from build123d import *

# Parameters (mm, degrees)
ESQUISSE1_W                                       = 17
ESQUISSE1_H                                       = 40
BOSS_EXTRU_1_DEPTH                                = 4
CHAMBRAGE_POUR_VIS_SIX_PANS_CREUX_M21_D           = 2.4
CHAMBRAGE_POUR_VIS_SIX_PANS_CREUX_M21_CBORE_D     = 4.4
CHAMBRAGE_POUR_VIS_SIX_PANS_CREUX_M21_CBORE_DEPTH = 2.4
ESQUISSE7_W                                       = 12
ESQUISSE7_H                                       = 2.3
ESQUISSE7_W_2                                     = 2.3
ESQUISSE7_H_2                                     = 15
ENL_V_MAT_EXTRU_1_DEPTH                           = 1.2


with BuildPart() as part:
    # Esquisse1 → Boss.-Extru.1 (new body)
    with BuildSketch(Plane.XY):
        with Locations((1.5, 2.5)):
            Rectangle(ESQUISSE1_W, ESQUISSE1_H)
    extrude(amount=BOSS_EXTRU_1_DEPTH)

    # Chambrage pour vis à six pans creux M21 (through all)
    with Locations(Plane.XY.offset(4)):
        with Locations((4, -15), (4, 20)):
            CounterBoreHole(CHAMBRAGE_POUR_VIS_SIX_PANS_CREUX_M21_D / 2, CHAMBRAGE_POUR_VIS_SIX_PANS_CREUX_M21_CBORE_D / 2, CHAMBRAGE_POUR_VIS_SIX_PANS_CREUX_M21_CBORE_DEPTH)

    # Esquisse7 → Enlèv. mat.-Extru.1 (cut)
    with BuildSketch(Plane(origin=(0, 0, 0), x_dir=(-1, 0, 0), z_dir=(0, 0, -1))):
        with Locations((-4, -6)):
            Rectangle(ESQUISSE7_W, ESQUISSE7_H)
        with Locations((-4, 10)):
            Rectangle(ESQUISSE7_W_2, ESQUISSE7_H_2)
    extrude(amount=-ENL_V_MAT_EXTRU_1_DEPTH, mode=Mode.SUBTRACT)


solid = part.part
Part model, mm, in its own coordinate system. A direction names the side the tool comes from. Give positions to 0.01 mm unless a question says otherwise; leave off trailing zeros. Order: outer loops, then holes, each group sorted by start corner. A loop starts at its lowest first (then second) coordinate and runs counter-clockwise, first axis right, second up. Notation, with made-up numbers: (10, 53.25) - (32, 53.25) arc R19 ccw to (32, 81.25) - close; hole circle Ø1 at (29.25, -40). An arc over 180 degrees is marked (long way). Use a Markdown table: item, result.
1) Saw through at D-D on z = 2.65. List the corners of the cut face in (x, y), plus the area to 3 significant figures.
Checked values:
| item | result |
|---|---|
| outline | (-7, -17.5) - (10, -17.5) - (10, 22.5) - (-7, 22.5) - close; hole circle Ø4.4 at (4, -15); hole circle Ø4.4 at (4, 20) |
| area | 650 mm² |
2) Two-plate mould, pull along X, no slides. Class faces 6 (the flat face through (1, 3, 0)), 7 (the flat face through (5, 19, 1.6)), 8 (the flat face through (10, 2, 2)): +X half, -X half, draft (parallel to the pull), parting line (faces both ways), or undercut.
Checked values:
| item | result |
|---|---|
| face 6 | draft |
| face 7 | undercut |
| face 8 | +X half |
3) Saw through at C-C on x = 0.25. List the corners of the cut face in (y, z), plus the area to 3 significant figures.
Checked values:
| item | result |
|---|---|
| outline | (-17.5, 0) - (-7.15, 0) - (-7.15, 1.2) - (-4.85, 1.2) - (-4.85, 0) - (22.5, 0) - (22.5, 4) - (-17.5, 4) - close |
| area | 157 mm² |
4) Flat gauge pins, fed straight in: P1, Ø0.7, axis at x = 4.5, y = -6.5, coming from the -Z side; P2, Ø2, axis at x = 3, y = -14, coming from the +Z side; P3, Ø2, axis at x = 4, y = -15, coming from the +Z side; P4, Ø2, axis at x = 5, y = 20.5, coming from the +Z side. Where does each tip first touch, or does it go through?
Checked values:
| item | result |
|---|---|
| P1 | z = 1.2 |
| P2 | z = 4 |
| P3 | through |
| P4 | z = 1.6 |
5) Saw through at B-B on x = 4. List the corners of the cut face in (y, z).
Checked values:
| item | result |
|---|---|
| outline | (-17.5, 0) - (-16.2, 0) - (-16.2, 1.6) - (-17.2, 1.6) - (-17.2, 4) - (-17.5, 4) - close; (-13.8, 0) - (-7.15, 0) - (-7.15, 1.2) - (-4.85, 1.2) - (-4.85, 0) - (2.5, 0) - (2.5, 1.2) - (17.5, 1.2) - (17.5, 0) - (18.8, 0) - (18.8, 1.6) - (17.8, 1.6) - (17.8, 4) - (-12.8, 4) - (-12.8, 1.6) - (-13.8, 1.6) - close; (21.2, 0) - (22.5, 0) - (22.5, 4) - (22.2, 4) - (22.2, 1.6) - (21.2, 1.6) - close |
6) Probe L1, parallel to Y at x = 4, z = 0.3; L2, parallel to Y at x = 9.25, z = 0.2; L3, parallel to Y at x = 4, z = 2.7. List the from-to ranges inside material, lowest first. Write a range as from..to.
Checked values:
| item | result |
|---|---|
| L1 | -17.5..-16.2, -13.8..-7.15, -4.85..2.5, 17.5..18.8, 21.2..22.5 |
| L2 | -17.5..-7.15, -4.85..22.5 |
| L3 | -17.5..-17.2, -12.8..17.8, 22.2..22.5 |
7) Saw through at A-A on y = -15. List the corners of the cut face in (x, z).
Checked values:
| item | result |
|---|---|
| outline | (-7, 0) - (2.8, 0) - (2.8, 1.6) - (1.8, 1.6) - (1.8, 4) - (-7, 4) - close; (5.2, 0) - (10, 0) - (10, 4) - (6.2, 4) - (6.2, 1.6) - (5.2, 1.6) - close |
8) 3-axis set-ups, long thin cutter, end or side, ignore diameter. For faces 1 (the flat face through (4, -6, 1.2)), 2 (the flat face through (2.85, 10, 1)), 3 (the flat face through (1, 22.5, 2)), 4 (the cylindrical face through (4.26, 18.83, 0.79)), 5 (the cylindrical face through (3.523, 17.852, 2.817)): which of +Z, -Z, +X, -X, +Y, -Y reach the whole face in a straight line?
Checked values:
| item | result |
|---|---|
| face 1 | -Z, +X |
| face 2 | -Z |
| face 3 | +Z, -Z, +X, -X, +Y |
| face 4 | +Z, -Z |
| face 5 | +Z |
